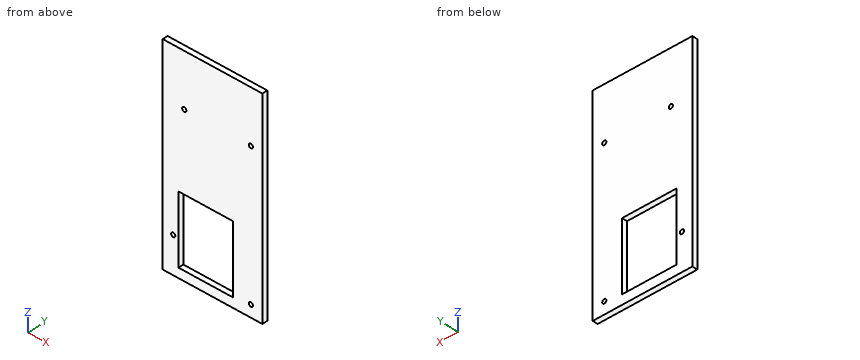
```python
from build123d import *

# Parameters (mm, degrees)
F0_W     = 95
F0_H     = 199.22458
F0_R     = 2
F0_W_2   = 52
F0_H_2   = 65.903932
F1_DEPTH = 5


with BuildPart() as f1:
    # F0 (on Front) → F1 (new body)
    with BuildSketch(Plane.XZ):
        with Locations((42.5, 94.61229)):
            Rectangle(F0_W, F0_H)
        with Locations((5, 30)):
            Circle(F0_R, mode=Mode.SUBTRACT)
        with Locations((36, 37.048034)):
            Rectangle(F0_W_2, F0_H_2, mode=Mode.SUBTRACT)
        with Locations((79, 6.5)):
            Circle(F0_R, mode=Mode.SUBTRACT)
        with Locations((15.5, 143.5)):
            Circle(F0_R, mode=Mode.SUBTRACT)
        with Locations((79, 143.5)):
            Circle(F0_R, mode=Mode.SUBTRACT)
    extrude(amount=F1_DEPTH)


solid = f1.part
```
The listing builds one solid part. Answer for the finished solid, in the listing's coordinates (mm). Coordinates: 2 decimals unless noted, no trailing zeros. Order: outer loops, then holes, each group sorted by start corner. A loop starts at its lowest first (then second) coordinate and runs counter-clockwise, first axis right, second up. Notation, with made-up numbers: M 32.5,-20 L 67.5,-20 A11 cw 67.5,-12 Z; hole C 4.25,-39.5 d6. An arc over 180 degrees is marked long. Answer as a JSON object with one key per item and string values. Group by question number.
1. Section B-B on z = 143.5 is taken. Write down the section's boundary in (x, y).
2. Section A-A on x = 15.5 is taken. Write down the section's boundary in (y, z), then the cut area to 3 significant figures.
3. Section C-C on y = -2.45 is taken. Write down the section's boundary in (x, z).
4. Straight lines are drawn through the part: line 1 (Z direction, x = 79, y = -3.3); line 2 (Z direction, x = 15.5, y = -1.95); line 3 (Z direction, x = 5, y = -0.95). For each, find the intervals that lie inside material, in ascending order.
5. Section D-D on x = 5 is taken. Write down the section's boundary in (y, z).
Values follow:
{
 "1": {"outline": "M -5,-5 L 13.5,-5 L 13.5,0 L -5,0 Z; M 17.5,-5 L 77,-5 L 77,0 L 17.5,0 Z; M 81,-5 L 90,-5 L 90,0 L 81,0 Z"},
 "2": {"outline": "M -5,-5 L 0,-5 L 0,4.1 L -5,4.1 Z; M -5,70 L 0,70 L 0,141.5 L -5,141.5 Z; M -5,145.5 L 0,145.5 L 0,194.22 L -5,194.22 Z", "area": "647 mm2"},
 "3": {"outline": "M -5,-5 L 90,-5 L 90,194.22 L -5,194.22 Z; hole C 5,30 d4; hole M 10,4.1 L 62,4.1 L 62,70 L 10,70 Z; hole C 15.5,143.5 d4; hole C 79,6.5 d4; hole C 79,143.5 d4"},
 "4": {"line 1": "-5 to 4.5, 8.5 to 141.5, 145.5 to 194.22", "line 2": "-5 to 4.1, 70 to 141.5, 145.5 to 194.22", "line 3": "-5 to 28, 32 to 194.22"},
 "5": {"outline": "M -5,-5 L 0,-5 L 0,28 L -5,28 Z; M -5,32 L 0,32 L 0,194.22 L -5,194.22 Z"}
}
